Geometry: see drawing. Coordinates: mm, zero at the bounding-box minimum. A direction names the side the tool comes from. Round coordinates to 2 decimals unless told otherwise and drop trailing zeros. Write each loop counter-clockwise with the first axis right and the second up, starting at its lowest first coordinate (ties: lowest second). Pieces come first, ordered by that corner, then holes.
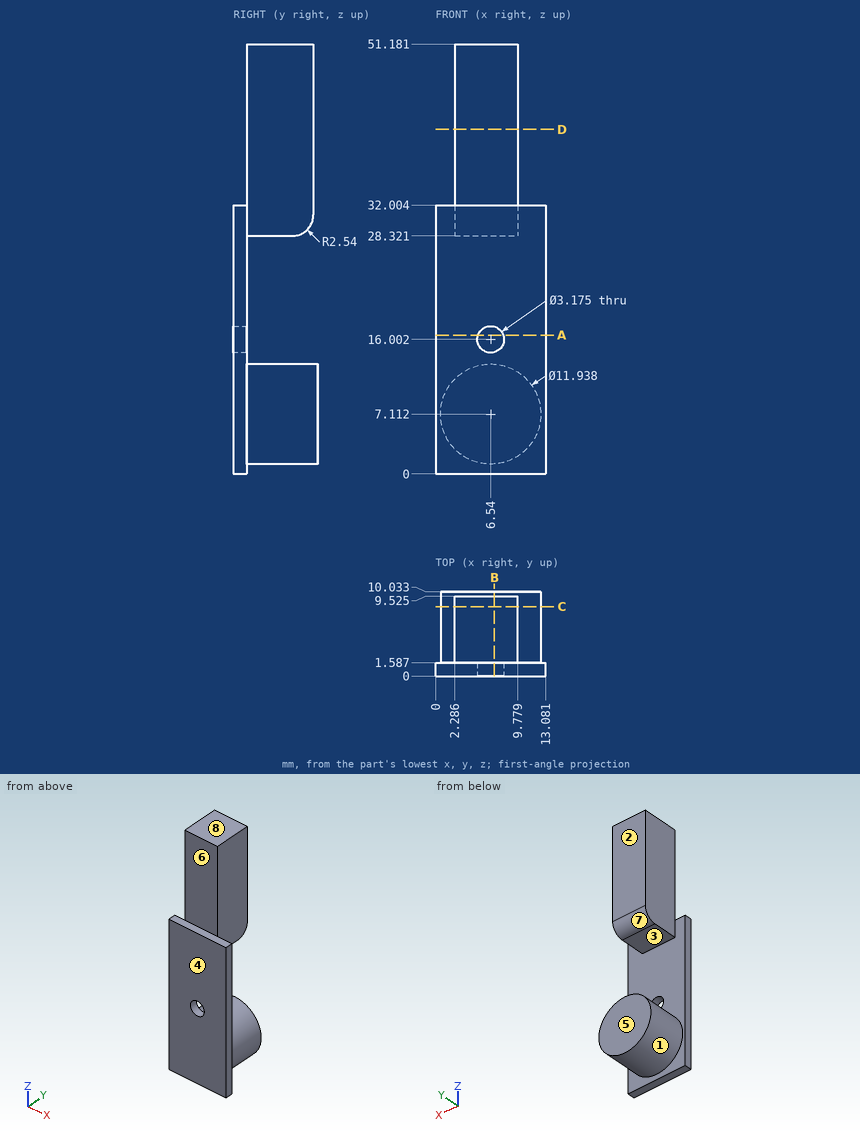
1) Pull-direction query (Z, two-part tool) for the marked faces 6, 7 and 8; classes: released by +Z, released by -Z, zero draft, split by the parting line, or undercut.
Taken from the geometry:
face 6: zero draft
face 7: undercut
face 8: released by +Z
2) Section query B-B on x = 7. Return the cut outline in (y, z) (1 decimal).
Taken from the geometry:
outline: (0, 0) - (1.6, 0) - (1.6, 1.2) - (10, 1.2) - (10, 13.1) - (1.6, 13.1) - (1.6, 14.5) - (0, 14.5) - close; (0, 17.5) - (1.6, 17.5) - (1.6, 28.3) - (7, 28.3) arc R2.5 ccw to (9.5, 30.9) - (9.5, 51.2) - (1.6, 51.2) - (1.6, 32) - (0, 32) - close
3) Reachability of the marked faces 1, 2, 3, 4 and 5 from +Z, -Z, +X, -X, +Y, -Y: full face, straight path, thin tool, end or side. Return the list, or none.
Taken from the geometry:
face 1: +Y
face 2: +Z, +X, -X, +Y
face 3: +X, -X, +Y
face 4: +Z, -Z, +X, -X, -Y
face 5: +Z, -Z, +X, -X, +Y
4) Section query A-A on z = 16.5. Return the cut outline in (x, y).
Taken from the geometry:
outline: (0, 0) - (5.03, 0) - (5.03, 1.59) - (0, 1.59) - close; (8.05, 0) - (13.08, 0) - (13.08, 1.59) - (8.05, 1.59) - close
5) Section query D-D on z = 41. Return the cut outline in (x, y) (1 decimal).
Taken from the geometry:
outline: (2.3, 1.6) - (9.8, 1.6) - (9.8, 9.5) - (2.3, 9.5) - close
6) Contact query for flat-ended pins moving along their axis: P1, Ø1.5, axis at x = 2.5, z = 21.5, coming from the -Y side; P2, Ø2.5, axis at x = 5.5, y = 5, coming from the -Z side; P3, Ø3, axis at y = 6.5, z = 39, coming from the +X side; P4, Ø2, axis at y = 5.5, z = 12, coming from the -X side. Output: stop coordinate, or through.
Taken from the geometry:
P1: stops at y = 0
P2: stops at z = 1.14
P3: stops at x = 9.78
P4: stops at x = 2.01
7) Material intervals for line 1 (Y direction, x = 9.5, z = 43) (1 decimal); line 2 (X direction, y = 3.25, z = 47) (1 decimal); line 3 (Y direction, x = 10, z = 16.5), sorted ascending.
Taken from the geometry:
line 1: y = 1.6 to 9.5
line 2: x = 2.3 to 9.8
line 3: y = 0 to 1.59
8) Section query C-C on y = 8.25. Return the cut outline in (x, z) (1 decimal).
Taken from the geometry:
outline: circle Ø11.9 at (6.5, 7.1); (2.3, 28.7) - (9.8, 28.7) - (9.8, 51.2) - (2.3, 51.2) - close
